Autodesk Inventor part; units mm, degrees
ref_plane "YZ Plane" through (0, 0, 0) normal (1, 0, 0) x (0, 1, 0)
ref_plane "XZ Plane" through (0, 0, 0) normal (0, 1, 0) x (-1, 0, 0)
ref_plane "XY Plane" through (0, 0, 0) normal (0, 0, 1) x (1, 0, 0)
sketch "Sketch1" plane through (0, 0, 0) normal (0, 0, 1) x (1, 0, 0)
  circle A0 centre (0, 0) radius 2.5
  dimension "Diameter" = 5
extrude "Extrusion1" add sketch "Sketch1" along normal blind 6.9
sketch "Sketch2" plane through (0, 0, 6.9) normal (0, 0, 1) x (1, 0, 0)
  circle A0 centre (0, 0) radius 2.5
extrude "Extrusion2" add sketch "Sketch2" along normal blind 3.1 draft 45
sketch "Sketch3" plane through (0, 0, 10) normal (0, 0, 1) x (1, 0, 0)
  circle A0 centre (0, 0) radius 5.6
  circle A1 centre (0, 0) radius 1.7321 construction
  line L0 (0.725, 1.573) -> (1.7248, 0.1586)
  line L1 (1.7248, 0.1586) -> (0.9997, -1.4144)
  line L2 (0.9997, -1.4144) -> (-0.725, -1.573)
  line L3 (-0.725, -1.573) -> (-1.7248, -0.1586)
  line L4 (-1.7248, -0.1586) -> (-0.9997, 1.4144)
  line L5 (-0.9997, 1.4144) -> (0.725, 1.573)
  dimension "Hex_Width" = 3
extrude "Extrusion3" cut sketch "Sketch3" against normal blind 2 contours L0 L1 L2 L3 L4 L5
thread "Thread1"
chamfer "Chamfer2" distance 0.5 angle 45 1 edges at (-2.5, 0, 0)
fillet "Fillet1" radius 0.1 1 edges at (-5.6, 0, 10)
equation "\"d10\" = Thread_Length"
equation "\"d13\" = Chamfer"
equation "\"Thread_Length\" = 6.9"
properties part number "SCREW, FLAT HD, P, 5, M5X0_8X10MM"
The listing builds one solid part. Answer for the finished solid, in the listing's coordinates (mm). A direction names the side the tool comes from. Give positions to 0.01 mm unless a question says otherwise; leave off trailing zeros. Loops run counter-clockwise (first coordinate to the right, second up) from the corner with the lowest first, then second, coordinate; pieces in that order, holes last. Notation, with made-up numbers: M 17,15 L 30,15 A18 cw 30,30 Z; hole C 29,0.5 d5. An arc over 180 degrees is marked long. Answer as CSV lines item,"result".
Item 1: Straight lines are drawn through the part: line 1 along Z through (x, y) = (1, -0.75); line 2 along Y through (x, z) = (3.5, 9); line 3 along X through (y, z) = (-2, 7). For each, find the intervals that lie inside material, in ascending order. Write a range as [from, to].
Values follow:
line 1,"z = [0, 8]"
line 2,"y = [-2.98, 2.98]"
line 3,"x = [-1.66, 1.66]"
Item 2: The mould has two halves that part along X. Classify faces 1 (the cylindrical face through (-0.54, 2.44, 3.66)), 2 (the flat face through (-1.3, -1.1, 10)), 3 (the flat face through (0.149, -1.493, 9.014)): released by +X, released by -X, zero draft, split by the parting line, or undercut.
Values follow:
face 1,"split by the parting line"
face 2,"zero draft"
face 3,"undercut"
Item 3: Given pin 1 Ø3 at (x, y) = (3, -4) entering from -Z; pin 2 Ø4 at (y, z) = (-2, 2) entering from +X; pin 3 Ø2 at (y, z) = (1.5, 7.5) entering from -X; pin 4 Ø1 at (y, z) = (4, 7) entering from -X, each flat-ended and moving along its own axis, determine where each tip first touches the part or whether it passes through.
Values follow:
pin 1,"stops at z = 7.9"
pin 2,"stops at x = 2.5"
pin 3,"stops at x = -3.87"
pin 4,"passes through"
Item 4: Which of the six approach directions +Z, -Z, +X, -X, +Y, -Y give full straight-line access (tool end or side, diameter ignored) to faces 4 (the flat face through (0, 0, 0)), 5 (the flat face through (-1.367, 0.617, 9.014))?
Values follow:
face 4,"-Z, +X, -X, +Y, -Y"
face 5,"+Z"
Item 5: The part is cut by section C-C (y = 0). Give the vertices of the cut face in (x, z), and give its area (3 significant figures).
Values follow:
outline,"M -5.43,9.83 L -2.5,6.9 L -2.5,0.5 L -2,0 L 2,0 L 2.5,0.5 L 2.5,6.9 L 5.43,9.83 A0.1 ccw 5.36,10 L 1.65,10 L 1.65,8 L -1.65,8 L -1.65,10 L -5.36,10 A0.1 ccw Z"
area,"52.7 mm^2"
Item 6: The part is cut by section B-B (x = 0). Give the vertices of the cut face in (y, z), and give its area (3 significant figures).
Values follow:
outline,"M -5.43,9.83 L -2.5,6.9 L -2.5,0.5 L -2,0 L 2,0 L 2.5,0.5 L 2.5,6.9 L 5.43,9.83 A0.1 ccw 5.36,10 L 1.51,10 L 1.51,8 L -1.51,8 L -1.51,10 L -5.36,10 A0.1 ccw Z"
area,"53.3 mm^2"
Item 7: The part is cut by section A-A (z = 4.25). Give the vertices of the cut face in (x, y), and give its area (3 significant figures).
Values follow:
outline,"C 0,0 d5"
area,"19.6 mm^2"
